The model under review builds one solid part; all positions refer to its coordinate system, in mm. Face numbers are marked on the shaded views. A direction names the side the tool comes from. Coordinates: 2 decimals unless noted, no trailing zeros. Write each loop counter-clockwise with the first axis right and the second up, starting at its lowest first coordinate (ties: lowest second). Pieces come first, ordered by that corner, then holes. Notation, with made-up numbers: (72, 9) -> (76, 9) arc R15 ccw to (76, 13) -> close; hole circle Ø2 at (-36.75, 85). An arc over 180 degrees is marked (long way). Write each question's results on one line, items separated by ' | '.
```python
from build123d import *

# Parameters (mm, degrees)
BOSS_EXTRUDE1_DEPTH              = 7.62
CUT_EXTRUDE1_DEPTH               = 30.441514138
SKETCH3_W                        = 12.7
SKETCH3_H                        = 7.62
F_5_CLEARANCE_HOLE1_D            = 3.556
F_36_0_1065_DIAMETER_HOLE1_D     = 2.7051
F_36_0_1065_DIAMETER_HOLE1_DEPTH = 5.08
F_5_CLEARANCE_HOLE2_D            = 3.556
F_5_CLEARANCE_HOLE2_DEPTH        = 22.995384182


with BuildPart() as part:
    # Sketch1 → Boss-Extrude1 (new body)
    with BuildSketch(Plane(origin=(0, 7.62, 0), x_dir=(1, 0, 0), z_dir=(0, 1, 0))):
        with BuildLine():
            Line((23.057960451, -6.35), (23.057960451, 6.35))
            Line((23.057960451, 6.35), (17.227118157, 6.35))
            ThreePointArc((17.227118157, 6.35), (15.786457002, 6.695667846), (14.659490486, 7.657404449))
            ThreePointArc((14.659490486, 7.657404449), (14.589471792, 9.508848608), (15.564771332, 11.084138707))
            ThreePointArc((15.564771332, 11.084138707), (15.715448212, 15.715448212), (11.084138707, 15.564771332))
            ThreePointArc((11.084138707, 15.564771332), (9.317430783, 14.545190239), (7.295007228, 14.810907114))
            ThreePointArc((7.295007228, 14.810907114), (0, 16.51), (-7.295007228, 14.810907114))
            ThreePointArc((-7.295007228, 14.810907114), (-9.317430783, 14.545190239), (-11.084138707, 15.564771332))
            ThreePointArc((-11.084138707, 15.564771332), (-15.715448212, 15.715448212), (-15.564771332, 11.084138707))
            ThreePointArc((-15.564771332, 11.084138707), (-14.545190239, 9.317430783), (-14.810907114, 7.295007228))
            ThreePointArc((-14.810907114, 7.295007228), (-16.51, 0), (-14.810907114, -7.295007228))
            ThreePointArc((-14.810907114, -7.295007228), (-14.545190239, -9.317430783), (-15.564771332, -11.084138707))
            ThreePointArc((-15.564771332, -11.084138707), (-15.715448212, -15.715448212), (-11.084138707, -15.564771332))
            ThreePointArc((-11.084138707, -15.564771332), (-9.317430783, -14.545190239), (-7.295007228, -14.810907114))
            ThreePointArc((-7.295007228, -14.810907114), (0, -16.51), (7.295007228, -14.810907114))
            ThreePointArc((7.295007228, -14.810907114), (9.317430783, -14.545190239), (11.084138707, -15.564771332))
            ThreePointArc((11.084138707, -15.564771332), (15.715448212, -15.715448212), (15.564771332, -11.084138707))
            ThreePointArc((15.564771332, -11.084138707), (14.589471792, -9.508848608), (14.659490486, -7.657404449))
            ThreePointArc((14.659490486, -7.657404449), (15.786457002, -6.695667846), (17.227118157, -6.35))
            Line((17.227118157, -6.35), (23.057960451, -6.35))
        make_face()
    extrude(amount=-BOSS_EXTRUDE1_DEPTH)

    # Sketch2 → Cut-Extrude1 (cut, through all)
    with BuildSketch(Plane.XZ):
        with BuildLine():
            Line((23.057960451, -1.27), (23.057960451, 1.27))
            Line((23.057960451, 1.27), (12.636340451, 1.27))
            ThreePointArc((12.636340451, 1.27), (12.7, 0), (12.636340451, -1.27))
            Line((12.636340451, -1.27), (23.057960451, -1.27))
        make_face()
    extrude(amount=-CUT_EXTRUDE1_DEPTH, mode=Mode.SUBTRACT)

    # Sketch3 → Cut-Revolve1 (revolve, cut)
    with BuildSketch(Plane.XY):
        with Locations((6.35, 3.81)):
            Rectangle(SKETCH3_W, SKETCH3_H)
    revolve(axis=Axis((0, 7.62, 0), (0, -1, 0)), mode=Mode.SUBTRACT)

    # #5 Clearance Hole1 (through all)
    with Locations(Plane(origin=(0, 7.62, 0), x_dir=(1, 0, 0), z_dir=(0, 1, 0))):
        with Locations((13.470384182, -13.470384182), (-13.470384182, -13.470384182), (-13.470384182, 13.470384182), (13.470384182, 13.470384182)):
            Hole(F_5_CLEARANCE_HOLE1_D / 2)

    # #36 (0.1065) Diameter Hole1
    with Locations(Plane(origin=(0, 0, -6.35), x_dir=(-1, 0, 0), z_dir=(0, 0, -1))):
        with Locations((-19.438793191, 3.81)):
            Hole(F_36_0_1065_DIAMETER_HOLE1_D / 2, depth=F_36_0_1065_DIAMETER_HOLE1_DEPTH)

    # #5 Clearance Hole2
    with Locations(Plane.XY.offset(6.35)):
        with Locations((19.438793191, 3.81)):
            Hole(F_5_CLEARANCE_HOLE2_D / 2, depth=F_5_CLEARANCE_HOLE2_DEPTH)


solid = part.part
```
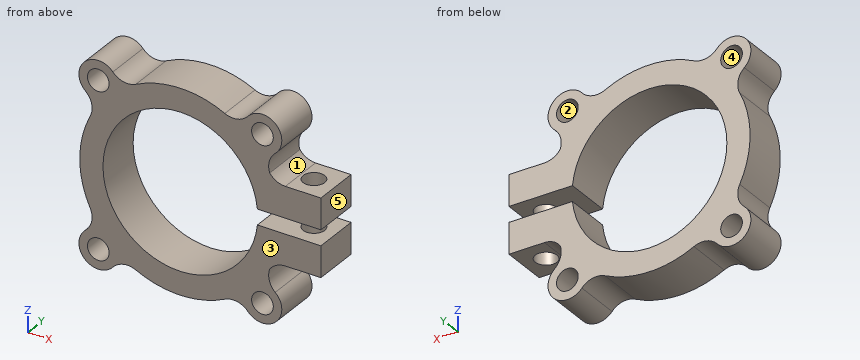
Q1. Add section B-B (z = 5). Write out the cut boundary in (x, y).
Solution:
outline: (-15.73, 0) -> (-11.67, 0) -> (-11.67, 7.62) -> (-15.73, 7.62) -> close; (11.67, 0) -> (23.06, 0) -> (23.06, 7.62) -> (11.67, 7.62) -> close; hole circle Ø3.56 at (19.44, 3.81)
Q2. Draft analysis for pull direction X (two halves, no side actions). For the marked faces 3, 4 and 5, state which applies: pulls with the +X half, pulls with the -X half, needs draft (parallel to the pull), parting line crosses it, or undercut.
Solution:
face 3: needs draft | face 4: undercut | face 5: pulls with the +X half
Q3. Add section A-A (x = 0). Write out the cut boundary in (y, z).
Solution:
outline: (0, -16.51) -> (7.62, -16.51) -> (7.62, -12.7) -> (0, -12.7) -> close; (0, 12.7) -> (7.62, 12.7) -> (7.62, 16.51) -> (0, 16.51) -> close
Q4. Clearance check with flat-ended pins moving along their axes: P1, Ø1, axis at x = -11, y = 3.5, coming from the +Z side; P2, Ø2, axis at x = 19.44, y = 3.81, coming from the +Z side; P3, Ø3, axis at x = 7, y = 2.5, coming from the +Z side; P4, Ø4.5, axis at x = 21, y = 2, coming from the +Z side. State where each tip first meets the part, or that it passes through.
Solution:
P1: z = 15.96 | P2: through | P3: z = 15.57 | P4: z = 6.35
Q5. Add section D-D (z = -14). Write out the cut boundary in (x, y), plus the area to 3 significant figures.
Solution:
outline: (-16.6, 0) -> (-15.17, 0) -> (-15.17, 7.62) -> (-16.6, 7.62) -> close; (-11.77, 0) -> (11.77, 0) -> (11.77, 7.62) -> (-11.77, 7.62) -> close; (15.17, 0) -> (16.6, 0) -> (16.6, 7.62) -> (15.17, 7.62) -> close | area: 201 mm²
Q6. Add section C-C (y = 1). Count the separate pieces of the cut face and the enclosed holes in it, plus the area to 3 significant figures.
Solution:
separate pieces: 1 | enclosed holes: 4 | area: 512 mm²
Q7. For line 1 (X direction, y = 2.25, z = -13.5); line 2 (X direction, y = 3, z = -3); line 3 (Z direction, x = 18.5, y = 1.75), list the stretches that pass through material, from the lowest coordinate up. Write a range as from..to.
Solution:
line 1: -16.65..-15.25, -11.69..11.69, 15.25..16.65 | line 2: -16.24..-12.34, 12.34..17.86, 21.02..23.06 | line 3: -6.35..-1.27, 1.27..6.35
Q8. Machinability: for the marked faces 1 and 2, which of the approach directions +Z, -Z, +X, -X, +Y, -Y give a long, thin tool a straight path to every point of the face, cutting with its end or side? Answer none if there is none.
Solution:
face 1: +X, +Y, -Y | face 2: +Y, -Y
